Part model, mm, in its own coordinate system. Face numbers are marked on the shaded views. A direction names the side the tool comes from. Round coordinates to 2 decimals unless told otherwise and drop trailing zeros. Write each loop counter-clockwise with the first axis right and the second up, starting at its lowest first coordinate (ties: lowest second). Pieces come first, ordered by that corner, then holes. Notation, with made-up numbers: (-22, 1.25) -> (5, 1.25) arc R18 ccw to (5, 30.25) -> close; hole circle Ø9 at (-6, 1). An arc over 180 degrees is marked (long way). Return JSON: item names as keys, results as strings. Group by question number.
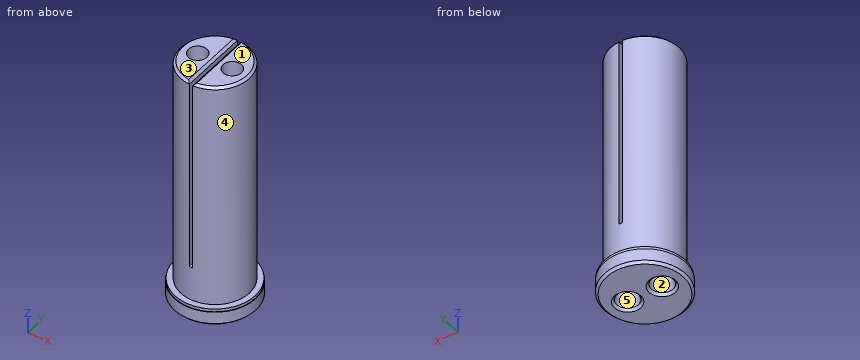
```python
from build123d import *

# Parameters (mm, degrees)
SKETCH014_R     = 7.05
PAD004_DEPTH    = 2.5
SKETCH015_R     = 6.95
PAD005_DEPTH    = 0.5
SKETCH016_R     = 5.95
PAD006_DEPTH    = 40
SKETCH018_R     = 1.9
POCKET010_DEPTH = 5
SKETCH019_R     = 1.6
POCKET011_DEPTH = 43.001
SKETCH020_W     = 0.6
SKETCH020_H     = 16
POCKET012_DEPTH = 34
CHAMFER_SIZE    = 0.4
CHAMFER003_SIZE = 0.4


with BuildPart() as part:
    # Sketch014 → Pad004 (new body)
    with BuildSketch(Plane.XY):
        Circle(SKETCH014_R)
    extrude(amount=PAD004_DEPTH)

    # Sketch015 (on DatumPlane) → Pad005 (join)
    with BuildSketch(Plane.XY.offset(2.5)):
        Circle(SKETCH015_R)
    extrude(amount=PAD005_DEPTH)

    # Sketch016 (on DatumPlane) → Pad006 (join)
    with BuildSketch(Plane.XY.offset(3)):
        Circle(SKETCH016_R)
    extrude(amount=PAD006_DEPTH)

    # Sketch018 (on DatumPlane) → Pocket010 (cut)
    with BuildSketch(Plane.XY):
        with Locations((-3, 0)):
            Circle(SKETCH018_R)
        with Locations((3, 0)):
            Circle(SKETCH018_R)
    extrude(amount=POCKET010_DEPTH, mode=Mode.SUBTRACT)

    # Sketch019 (on DatumPlane) → Pocket011 (cut, through all)
    with BuildSketch(Plane.XY):
        with Locations((-3, 0)):
            Circle(SKETCH019_R)
        with Locations((3, 0)):
            Circle(SKETCH019_R)
    extrude(amount=POCKET011_DEPTH, mode=Mode.SUBTRACT)

    # Sketch020 (on DatumPlane) → Pocket012 (cut)
    with BuildSketch(Plane.XY.offset(43)):
        Rectangle(SKETCH020_W, SKETCH020_H)
    extrude(amount=-POCKET012_DEPTH, mode=Mode.SUBTRACT)

    # Chamfer
    chamfer_edges = [part.edges().sort_by_distance(p)[0] for p in [
        (-0.3, 0, 43),
        (-5.95, 0, 43),
        (0.3, 0, 43),
        (4.312047, -4.099848, 43),
        (4.312047, 4.099848, 43),
    ]]
    chamfer(chamfer_edges, length=CHAMFER_SIZE)

    # Chamfer003
    chamfer003_edges = [part.edges().sort_by_distance(p)[0] for p in [
        (-7.05, 0, 0),
        (-4.9, 0, 0),
        (1.1, 0, 0),
    ]]
    chamfer(chamfer003_edges, length=CHAMFER003_SIZE)


with BuildPart() as part_1:
    # Body003 placement: moved
    add(part.part.moved(Location((0, 0, 22))))


solid = part_1.part
```
Item 1: Cut at A-A (z = 54.5). Write the cut outline in (x, y), then the cut area to 3 significant figures.
Item 2: Wall check: L1, parallel to X at y = 0, z = 39; L2, parallel to X at y = 1.25, z = 36.5; L3, parallel to Z at x = -0.75, y = -5.5. Give the ranges that are in metal, low to high.
Item 3: Which spindle directions (+Z, -Z, +X, -X, +Y, -Y) get a long thin tool onto all of the face, cutting with end or side? Do the marked faces 1 and 2. Say none if no direction does.
Item 4: Flat gauge pins, fed straight in: P1, Ø2, axis at y = -3, z = 39, coming from the -X side; P2, Ø0.5, axis at x = 0, y = -0.5, coming from the +Z side; P3, Ø8, axis at x = -0.5, z = 50.5, coming from the -Y side. Where does each tip first touch, or does it go through?
Item 5: Cut at B-B (y = 0). State how many separate pieces and enclosed holes the cut face has, then the cut area to 3 significant figures.
Item 6: Two-plate mould, pull along Y, no slides. Class the marked faces 3, 4 and 5: released by +Y, released by -Y, zero draft, split by the parting line, or undercut.
Checks:
{
 "1": {"outline": "(-0.3, -5.94) -> (-0.3, 5.94) arc R5.95 ccw to start; (0.3, -5.94) arc R5.95 ccw to (0.3, 5.94) -> close; hole circle Ø3.2 at (-3, 0); hole circle Ø3.2 at (3, 0)", "area": "88.0 mm2"},
 "2": {"L1": "x = -5.95 to -4.6, -1.4 to -0.3, 0.3 to 1.4, 4.6 to 5.95", "L2": "x = -5.82 to -4, -2 to -0.3, 0.3 to 2, 4 to 5.82", "L3": "z = 22 to 65"},
 "3": {"face 1": "+Z, +X, -X, +Y, -Y", "face 2": "-Z"},
 "4": {"P1": "stops at x = -5.6", "P2": "stops at z = 31", "P3": "stops at y = -5.94"},
 "5": {"separate pieces": "3", "enclosed holes": "0", "area": "216 mm2"},
 "6": {"face 3": "zero draft", "face 4": "split by the parting line", "face 5": "undercut"}
}
